from build123d import *

# Parameters (mm, degrees)
SKETCH1_R           = 1.5
BOSS_EXTRUDE1_DEPTH = 5


with BuildPart() as part:
    # Sketch1 → Boss-Extrude1 (new body)
    with BuildSketch(Plane.XY):
        Polygon((0, 0), (0, -25), (10, -25), (10, -20), (20, -10), (100, -10), (100, 0), align=None)
        with Locations((5, -20)):
            Circle(SKETCH1_R, mode=Mode.SUBTRACT)
        with Locations((5, -5)):
            Circle(SKETCH1_R, mode=Mode.SUBTRACT)
    extrude(amount=BOSS_EXTRUDE1_DEPTH)

    # Mirror1: part across plane


with BuildPart() as part_1:
    add(part.part)
    add(part.part.mirror(Plane(origin=(100, -10, 5), x_dir=(0, 0, 1), z_dir=(-1, 0, 0))))


solid = part_1.part
Read the model definition and answer for the solid it produces. Units are mm, in the model's axes. A direction names the side the tool comes from. Round coordinates to 2 decimals unless told otherwise and drop trailing zeros. Order: outer loops, then holes, each group sorted by start corner. A loop starts at its lowest first (then second) coordinate and runs counter-clockwise, first axis right, second up. Notation, with made-up numbers: (45, 6) - (101, 6) arc R10 cw to (101, 15) - close; hole circle Ø5 at (-40, -10). An arc over 180 degrees is marked (long way). Use one line per item in the form item = value. Start each with the question number.
(1) For faces 1 (the face through (200, -12, 2)), 2 (the face through (10, -23, 2)), determine the directions among +Z, -Z, +X, -X, +Y, -Y from which every point of the face is accessible in a straight line to the end or side of a thin tool.
(2) Determine the mould class of faces 3 (the face through (185, -15, 2)), 4 (the face through (15, -15, 2)), 5 (the face through (101, -7, 5)), 6 (the face through (0, -12, 2)) for opening direction X: +X half, -X half, draft (parallel to the pull), parting line (faces both ways), or undercut.
(3) Find the intervals of material crossed by line 1 along Y through (x, z) = (5, 2.45); line 2 along Y through (x, z) = (63, 0.55); line 3 along X through (y, z) = (-4, 4.35), in increasing order. Write a range as from..to.
(4) The part is cut by section B-B (x = 48). Give the vertices of the cut face in (y, z), then the cut area to 3 significant figures.
(5) The part is cut by section A-A (z = 3.3). Give the vertices of the cut face in (x, y).
Checked values:
q1.face_1 = +Z, -Z, +X, +Y, -Y
q1.face_2 = +Z, -Z, -Y
q2.face_3 = undercut
q2.face_4 = undercut
q2.face_5 = draft
q2.face_6 = -X half
q3.line_1 = -25..-21.5, -18.5..-6.5, -3.5..0
q3.line_2 = -10..0
q3.line_3 = 0..3.88, 6.12..193.88, 196.12..200
q4.outline = (-10, 0) - (0, 0) - (0, 5) - (-10, 5) - close
q4.area = 50.0 mm^2
q5.outline = (0, -25) - (10, -25) - (10, -20) - (20, -10) - (180, -10) - (190, -20) - (190, -25) - (200, -25) - (200, 0) - (0, 0) - close; hole circle Ø3 at (5, -20); hole circle Ø3 at (5, -5); hole circle Ø3 at (195, -20); hole circle Ø3 at (195, -5)
